```python
from build123d import *

# Parameters (mm, degrees)
EXTRU_MINCE1_DEPTH      = 13
EXTRU_MINCE1_DEPTH_BACK = 13
ESQUISSE2_R             = 4
ESQUISSE2_R_2           = 1.75
ENL_V_MAT_EXTRU_1_DEPTH = 47.454278597
ESQUISSE3_R             = 4
ESQUISSE3_R_2           = 1.6
ENL_V_MAT_EXTRU_2_DEPTH = 47.454278597
CHANFREIN1_SIZE         = 0.5
CONG_1_R                = 3


with BuildPart() as part:
    # Esquisse1 → Extru.-Mince1 (new, two sides: drawn at the far end of the back side and taken through both)
    with BuildSketch(Plane.XY.offset(-EXTRU_MINCE1_DEPTH_BACK)):
        with BuildLine():
            Line((33, 0), (4, 0))
            ThreePointArc((4, 0), (1.171572875, 1.171572875), (0, 4))
            Line((0, 4), (0, 33))
            Line((0, 33), (3, 33))
            Line((3, 33), (3, 4))
            ThreePointArc((3, 4), (3.292893219, 3.292893219), (4, 3))
            Line((4, 3), (33, 3))
            Line((33, 3), (33, 0))
        make_face()
    extrude(amount=EXTRU_MINCE1_DEPTH + EXTRU_MINCE1_DEPTH_BACK)

    # Esquisse2 → Enlèv. mat.-Extru.1 (cut, through all)
    with BuildSketch(Plane(origin=(0, 3, 0), x_dir=(1, 0, 0), z_dir=(0, 1, 0))):
        with Locations(Location((18, 0, 0), (0, 0, 270))):
            Circle(ESQUISSE2_R)
        with Locations(Location((10.858571571, 7, 0), (0, 0, 270))):
            Circle(ESQUISSE2_R_2)
        with Locations(Location((10.858571571, -7, 0), (0, 0, 90))):
            Circle(ESQUISSE2_R_2)
        with Locations(Location((25.141428429, -7, 0), (0, 0, 270))):
            Circle(ESQUISSE2_R_2)
        with Locations(Location((25.141428429, 7, 0), (0, 0, 90))):
            Circle(ESQUISSE2_R_2)
    extrude(amount=-ENL_V_MAT_EXTRU_1_DEPTH, mode=Mode.SUBTRACT)

    # Esquisse3 → Enlèv. mat.-Extru.2 (cut, through all)
    with BuildSketch(Plane(origin=(3, 0, 0), x_dir=(0, 0, -1), z_dir=(1, 0, 0))):
        with Locations((0, 20)):
            Circle(ESQUISSE3_R)
        with Locations((-8.5, 20)):
            Circle(ESQUISSE3_R_2)
        with Locations(Location((8.5, 20, 0), (0, 0, 180))):
            Circle(ESQUISSE3_R_2)
        with BuildLine():
            Line((13, 20), (15, 20))
            Line((15, 20), (15, 35))
            Line((15, 35), (-15, 35))
            Line((-15, 35), (-15, 20))
            Line((-15, 20), (-13, 20))
            ThreePointArc((-13, 20), (0, 33), (13, 20))
        make_face()
    extrude(amount=-ENL_V_MAT_EXTRU_2_DEPTH, mode=Mode.SUBTRACT)

    # Chanfrein1
    chanfrein1_edges = [part.edges().sort_by_distance(p)[0] for p in [
        (0, 20, -10.1),
        (0, 20, 10.1),
    ]]
    chamfer(chanfrein1_edges, length=CHANFREIN1_SIZE)

    # Congé1
    cong_1_edges = [part.edges().sort_by_distance(p)[0] for p in [
        (33, 1.5, 13),
        (33, 1.5, -13),
    ]]
    fillet(cong_1_edges, radius=CONG_1_R)


solid = part.part
```
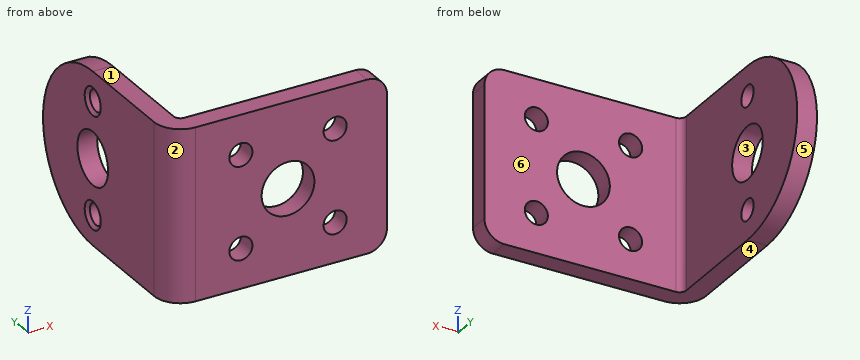
Geometry: final body of the model. Coordinates: model frame, mm. Face numbers are marked on the shaded views. A direction names the side the tool comes from. Give positions to 0.01 mm unless a question says otherwise; leave off trailing zeros. Order: outer loops, then holes, each group sorted by start corner. A loop starts at its lowest first (then second) coordinate and runs counter-clockwise, first axis right, second up. Notation, with made-up numbers: M 64,-36 L 73,-36 A22 ccw 73,-11 Z; hole C 76.25,-10.5 d3. An arc over 180 degrees is marked long. Answer as CSV lines item,"result". Start each with the question number.
1) Mould query, pull axis Z, two halves, no side actions, for the marked faces 1, 2, 3 and 4. Classes: +Z half, -Z half, draft (parallel to the pull), parting line (faces both ways), or undercut.
2) First-contact query: P1, Ø13, axis at x = 22.5, z = 4.5, coming from the +Y side; P2, Ø6, axis at y = 9, z = -5, coming from the +X side; P3, Ø1.5, axis at x = 28.5, z = -2.5, coming from the -Y side; P4, Ø3, axis at x = 25.14, z = -7, coming from the -Y side. Flat tips, straight axial feed; report the tip coordinate or a pass-through.
3) Cut plane A-A (z = 0). Output: boundary loops of the cut face in (x, y).
4) Cut plane D-D (y = 14.5). Output: boundary loops of the cut face in (x, z), then the cut area to 3 significant figures.
5) Line query: line 1 (X direction, y = 0.95, z = 7); line 2 (X direction, y = 1.15, z = 7); line 3 (Y direction, x = 12, z = -3.5). Output: solid intervals per line, ascending. Write a range as from..to.
6) Cut plane B-B (x = 18). Output: boundary loops of the cut face in (y, z).
7) Set-up query: the marked faces 5 and 6. Return all of +Z, -Z, +X, -X, +Y, -Y with unobstructed straight access to the full face (end or side cutting, diameter ignored); none if empty.
8) Cut plane C-C (x = 12). Output: boundary loops of the cut face in (y, z).
Findings below:
1,face 1,"+Z half"
1,face 2,"draft"
1,face 3,"undercut"
1,face 4,"-Z half"
2,P1,"stops at y = 3"
2,P2,"stops at x = 3"
2,P3,"stops at y = 0"
2,P4,"passes through"
3,outline,"M 0,4 A4 ccw 4,0 L 14,0 L 14,3 L 4,3 A1 cw 3,4 L 3,16 L 0,16 Z; M 0,24 L 3,24 L 3,33 L 0,33 Z; M 22,0 L 33,0 L 33,3 L 22,3 Z"
4,outline,"M 0,-13 L 3,-13 L 3,13 L 0,13 Z"
4,area,"78.0 mm²"
5,line 1,"x = 1.41..9.11, 12.61..23.39, 26.89..33"
5,line 2,"x = 1.19..9.11, 12.61..23.39, 26.89..33"
5,line 3,"y = 0..3"
6,outline,"M 0,-13 L 3,-13 L 3,-4 L 0,-4 Z; M 0,4 L 3,4 L 3,13 L 0,13 Z"
7,face 5,"+X, -X, +Y"
7,face 6,"+Z, -Z, +X, +Y"
8,outline,"M 0,-13 L 3,-13 L 3,-8.33 L 0,-8.33 Z; M 0,-5.67 L 3,-5.67 L 3,5.67 L 0,5.67 Z; M 0,8.33 L 3,8.33 L 3,13 L 0,13 Z"
